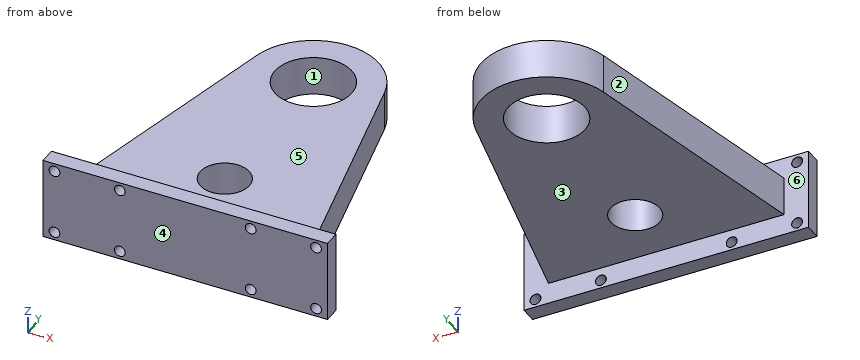
from build123d import *

# Parameters (mm, degrees)
SKETCH1_W                      = 174
SKETCH1_H                      = 50
BOSS_EXTRUDE1_DEPTH            = 10
M6_CLEARANCE_HOLE1_D           = 6.6
M6_CLEARANCE_HOLE1_CSINK_D     = 6.65
M6_CLEARANCE_HOLE1_CSINK_ANGLE = 100
BOSS_EXTRUDE2_DEPTH            = 12
BOSS_EXTRUDE2_DEPTH_BACK       = 12
CUT_EXTRUDE1_REACH             = 215.496
SKETCH7_R                      = 15
SKETCH7_R_2                    = 23.5


with BuildPart() as part:
    # Sketch1 → Boss-Extrude1 (new body)
    with BuildSketch(Plane(origin=(0, 0, 0), x_dir=(1, 0, 0), z_dir=(0, 1, 0))):
        Rectangle(SKETCH1_W, SKETCH1_H)
    extrude(amount=BOSS_EXTRUDE1_DEPTH)

    # M6 Clearance Hole1 (through all)
    with Locations(Plane(origin=(0, 10, 0), x_dir=(1, 0, 0), z_dir=(0, 1, 0))):
        with Locations((-80, 20), (-40, 20), (-80, -20), (-40, -20), (40, 20), (80, 20), (40, -20), (80, -20)):
            CounterSinkHole(M6_CLEARANCE_HOLE1_D / 2, M6_CLEARANCE_HOLE1_CSINK_D / 2, counter_sink_angle=M6_CLEARANCE_HOLE1_CSINK_ANGLE)

    # Sketch6 → Boss-Extrude2 (add, two sides: drawn at the far end of the back side and taken through both)
    with BuildSketch(Plane.XY.offset(-BOSS_EXTRUDE2_DEPTH_BACK)):
        with BuildLine():
            Line((-72, 10), (72, 10))
            Line((72, 10), (39.069577731, 160))
            ThreePointArc((39.069577731, 160), (0, 191.422815383), (-39.069577731, 160))
            Line((-39.069577731, 160), (-72, 10))
        make_face()
    extrude(amount=BOSS_EXTRUDE2_DEPTH + BOSS_EXTRUDE2_DEPTH_BACK)

    # Sketch7 → Cut-Extrude1 (cut, up to next)
    with BuildSketch(Plane.XY.offset(12), mode=Mode.PRIVATE) as cut_extrude1_sk1:
        with Locations((0, 46.722815383)):
            Circle(SKETCH7_R)
    cut_extrude1_tool1 = extrude(cut_extrude1_sk1.sketch, amount=-CUT_EXTRUDE1_REACH, mode=Mode.PRIVATE) & part.part
    # Sketch7 → Cut-Extrude1 (cut, up to next)
    with BuildSketch(Plane.XY.offset(12), mode=Mode.PRIVATE) as cut_extrude1_sk2:
        with Locations((0, 151.422815383)):
            Circle(SKETCH7_R_2)
    cut_extrude1_tool2 = extrude(cut_extrude1_sk2.sketch, amount=-CUT_EXTRUDE1_REACH, mode=Mode.PRIVATE) & part.part
    add(cut_extrude1_tool1.solids().sort_by_distance((0, 46.722815, 12))[0], mode=Mode.SUBTRACT)
    add(cut_extrude1_tool2.solids().sort_by_distance((0, 151.422815, 12))[0], mode=Mode.SUBTRACT)


solid = part.part
CAD build for the part. Positions are in the model's coordinates, mm. Face numbers are marked on the shaded views. A direction names the side the tool comes from. Round coordinates to 2 decimals unless told otherwise and drop trailing zeros. Loops run counter-clockwise (first coordinate to the right, second up) from the corner with the lowest first, then second, coordinate; pieces in that order, holes last. Notation, with made-up numbers: M 85.5,-10.5 L 116.5,-10.5 A23 ccw 116.5,23.5 Z; hole C -32,-9.5 d4. An arc over 180 degrees is marked long. One line per question, with ' | ' between items. Start each with the question number.
Item 1: Pin check, flat tips, straight feed: pin 1 Ø10.5 at (x, z) = (80, -20) entering from +Y; pin 2 Ø1 at (x, y) = (-40.5, 59.5) entering from -Z; pin 3 Ø5 at (y, z) = (67.5, -11) entering from -X. Stop position of each tip, or through.
Item 2: Cut at C-C, the plane z = 4.5. Write the cut outline in (x, y).
Item 3: Cut at B-B, the plane z = 20. Write the cut outline in (x, y) (3 decimals).
Item 4: Cut at A-A, the plane x = 0. Write the cut outline in (y, z).
Item 5: Two-plate mould, pull along X, no slides. Class the marked faces 1, 2 and 3: pulls with the +X half, pulls with the -X half, needs draft (parallel to the pull), parting line crosses it, or undercut.
Item 6: Wall check: line 1 (Z direction, x = -40, y = 5.25); line 2 (X direction, y = 5, z = 20); line 3 (Y direction, x = -21, z = -15). Give the ranges that are in metal, low to high.
Item 7: Which spindle directions (+Z, -Z, +X, -X, +Y, -Y) get a long thin tool onto all of the face, cutting with end or side? Do the marked faces 4, 5 and 6. Say none if no direction does.
Item 8: Cut at D-D, the plane x = -80. Write the cut outline in (y, z) (3 decimals).
Responses:
1) pin 1: stops at y = 10 | pin 2: stops at z = -12 | pin 3: stops at x = -59.93
2) outline: M -87,0 L 87,0 L 87,10 L 72,10 L 39.07,160 A40 ccw -39.07,160 L -72,10 L -87,10 Z; hole C 0,151.42 d47; hole C 0,46.72 d30
3) outline: M -87,0 L -83.3,0 L -83.3,9.979 L -83.325,10 L -87,10 Z; M -76.7,0 L -43.3,0 L -43.3,9.979 L -43.325,10 L -76.675,10 L -76.7,9.979 Z; M -36.7,0 L 36.7,0 L 36.7,9.979 L 36.675,10 L -36.675,10 L -36.7,9.979 Z; M 43.3,0 L 76.7,0 L 76.7,9.979 L 76.675,10 L 43.325,10 L 43.3,9.979 Z; M 83.3,0 L 87,0 L 87,10 L 83.325,10 L 83.3,9.979 Z
4) outline: M 0,-25 L 10,-25 L 10,-12 L 31.72,-12 L 31.72,12 L 10,12 L 10,25 L 0,25 Z; M 61.72,-12 L 127.92,-12 L 127.92,12 L 61.72,12 Z; M 174.92,-12 L 191.42,-12 L 191.42,12 L 174.92,12 Z
5) face 1: undercut | face 2: pulls with the -X half | face 3: needs draft
6) line 1: z = -25 to -23.3, -16.7 to 16.7, 23.3 to 25 | line 2: x = -87 to -83.3, -76.7 to -43.3, -36.7 to 36.7, 43.3 to 76.7, 83.3 to 87 | line 3: y = 0 to 10
7) face 4: +Z, -Z, +X, -X, -Y | face 5: +Z, +X, -X, +Y | face 6: +Y
8) outline: M 0,-25 L 10,-25 L 10,-23.325 L 9.979,-23.3 L 0,-23.3 Z; M 0,-16.7 L 9.979,-16.7 L 10,-16.675 L 10,16.675 L 9.979,16.7 L 0,16.7 Z; M 0,23.3 L 9.979,23.3 L 10,23.325 L 10,25 L 0,25 Z
